For this review, take the finished solid that the model builds, in its own axes (mm). Round coordinates to 2 decimals unless told otherwise and drop trailing zeros. Loops run counter-clockwise (first coordinate to the right, second up) from the corner with the lowest first, then second, coordinate; pieces in that order, holes last.
1) Take a section at A-A (x = 28). State the section outline as (y, z) points, then the cut area to 3 significant figures.
2) Insertion check: pin 1 (3 mm diameter, centred on x = 29, y = 2, fed in from +Z); pin 2 (1 mm diameter, centred on x = 37.5, z = 1, fed in from -Y); pin 3 (1 mm diameter, centred on x = 45.5, z = -2, fed in from -Y). Each pin has a flat end and moves straight along its axis. Give the tip position at first contact, or say it passes through.
3) Wall thickness on L1, parallel to X at y = -1.55, z = 2.4 (3 decimals); L2, parallel to Z at x = 3, y = -0.1; L3, parallel to Y at x = 33.5, z = 1.35: over which ranges is each line inside the solid? List them lowest first.
```python
from build123d import *

# Parameters (mm, degrees)
CHAMFER1_SIZE = 0.4


with BuildPart() as part:
    # Sketch1 → Revolve1 (revolve)
    with BuildSketch(Plane.XY):
        Polygon((-2, 0), (56.102, 0), (56.102, 3), (54.902, 3), (54.902, 2.667), (54.102, 2.667), (54.102, 3), (0, 3), (0, 2.667), (-0.8, 2.667), (-0.8, 3), (-2, 3), align=None)
    revolve(axis=Axis((-2, 0, 0), (-1, 0, 0)))

    # Chamfer1
    chamfer1_edges = [part.edges().sort_by_distance(p)[0] for p in [
        (-2, -3, 0),
        (56.102, -3, 0),
    ]]
    chamfer(chamfer1_edges, length=CHAMFER1_SIZE)


solid = part.part
```
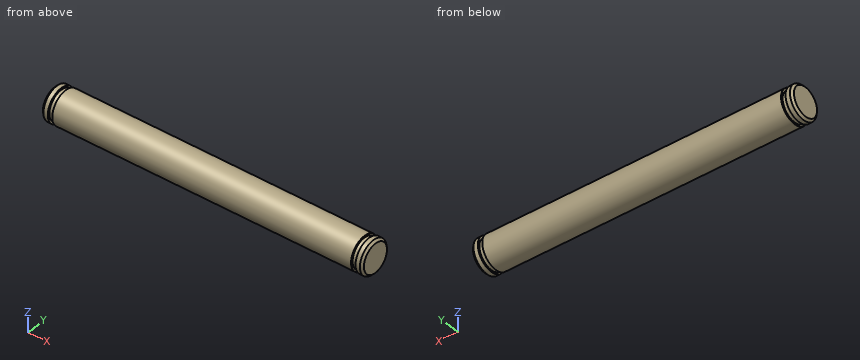
Response:
1. outline: circle Ø6 at (0, 0)
1. area: 28.3 mm2
2. pin 1: stops at z = 2.96
2. pin 2: stops at y = -2.96
2. pin 3: stops at y = -2.6
3. L1: x = -1.743 to -0.8, 0 to 54.102, 54.902 to 55.845
3. L2: z = -3 to 3
3. L3: y = -2.68 to 2.68
